Work out the finished part from the listing and answer in its coordinate system (mm). Face numbers are marked on the shaded views. A direction names the side the tool comes from. Coordinates: 2 decimals unless noted, no trailing zeros. Write each loop counter-clockwise with the first axis right and the second up, starting at its lowest first coordinate (ties: lowest second). Pieces come first, ordered by that corner, then holes. Notation, with made-up numbers: (22, 42.25) - (27, 42.25) arc R24 ccw to (27, 80.25) - close; hole circle Ø1 at (-8.5, -30.5). An arc over 180 degrees is marked (long way). One line per item, written item: value.
```python
from build123d import *

# Parameters (mm, degrees)
F1_DEPTH    = 8
F3_DEPTH    = 15
F4_T1_DEPTH = 8
F5_W        = 19.4
F5_H        = 25.4
F6_DEPTH    = 1.6
F7_W        = 17.4
F7_H        = 23.4
F8_DEPTH    = 25
F9_W        = 17.6963857411
F9_H        = 23.4
F10_DEPTH   = 5
F11_W       = 1
F11_H       = 16
F12_DEPTH   = 2


# Not quite as in the source:
# - a fillet or chamfer that OpenCascade refuses, or shapes differently, is made with other operations: its cross-section is extruded or revolved along the edge and cut away or added
# - a feature of the source that left no trace in its solid (it failed there, or was rolled back) is left out


with BuildPart() as f1:
    # F0 (on Front) → F1 (new body)
    with BuildSketch(Plane.XZ):
        with BuildLine():
            Line((5.123475383, -16.5), (14, -16.5))
            Line((14, -16.5), (14, 16.5))
            Line((14, 16.5), (5.123475383, 16.5))
            ThreePointArc((5.123475383, 16.5), (0, 14), (-5.123475383, 16.5))
            Line((-5.123475383, 16.5), (-14, 16.5))
            Line((-14, 16.5), (-14, -16.5))
            Line((-14, -16.5), (-5.123475383, -16.5))
            ThreePointArc((-5.123475383, -16.5), (0, -14), (5.123475383, -16.5))
        make_face()
    extrude(amount=F1_DEPTH)

    # F0 (on Front) → F3 (join)
    with BuildSketch(Plane.XZ):
        with BuildLine():
            ThreePointArc((6.5, -20.5), (6.1462423475, -18.3848865266), (5.123475383, -16.5))
            Line((5.123475383, -16.5), (1.4361406616, -16.5))
            ThreePointArc((1.4361406616, -16.5), (3.4760680238, -18.0547083826), (4.25, -20.5))
            ThreePointArc((4.25, -20.5), (-2.4452916174, -23.9760680238), (-1.4361406616, -16.5))
            Line((-1.4361406616, -16.5), (-5.123475383, -16.5))
            ThreePointArc((-5.123475383, -16.5), (-2.1151134734, -26.6462423475), (6.5, -20.5))
        make_face()
        with BuildLine():
            Line((1.4361406616, -16.5), (5.123475383, -16.5))
            ThreePointArc((5.123475383, -16.5), (0, -14), (-5.123475383, -16.5))
            Line((-5.123475383, -16.5), (-1.4361406616, -16.5))
            ThreePointArc((-1.4361406616, -16.5), (0, -16.25), (1.4361406616, -16.5))
        make_face()
        with BuildLine():
            ThreePointArc((-5.123475383, 16.5), (0, 14), (5.123475383, 16.5))
            Line((5.123475383, 16.5), (1.4361406616, 16.5))
            ThreePointArc((1.4361406616, 16.5), (0, 16.25), (-1.4361406616, 16.5))
            Line((-1.4361406616, 16.5), (-5.123475383, 16.5))
        make_face()
        with BuildLine():
            Line((1.4361406616, 16.5), (5.123475383, 16.5))
            ThreePointArc((5.123475383, 16.5), (6.1462423475, 18.3848865266), (6.5, 20.5))
            ThreePointArc((6.5, 20.5), (-2.1151134734, 26.6462423475), (-5.123475383, 16.5))
            Line((-5.123475383, 16.5), (-1.4361406616, 16.5))
            ThreePointArc((-1.4361406616, 16.5), (-2.4452916174, 23.9760680238), (4.25, 20.5))
            ThreePointArc((4.25, 20.5), (3.4760680238, 18.0547083826), (1.4361406616, 16.5))
        make_face()
    extrude(amount=F3_DEPTH)

    # F4: chamfer of 1.9 on 4 edges, made by hand

    # F4_s2 → F4_t1 (join)
    with BuildSketch(Plane.XZ):
        with BuildLine():
            Line((-6.8027454264, 16.4361025598), (-5.876418772, 17.87458352))
            Line((-5.876418772, 17.87458352), (-5.8418237692, 17.8903056629))
            ThreePointArc((-5.8418237692, 17.8903056629), (-5.5354543935, 17.1659051218), (-5.0935227577, 16.5233846154))
            Line((-5.0935227577, 16.5233846154), (-5.123475383, 16.462))
            ThreePointArc((-5.123475383, 16.462), (-5.9631104047, 16.462), (-6.8027454264, 16.3981025598))
            Line((-6.8027454264, 16.3981025598), (-6.8027454264, 16.4361025598))
        make_face()
        with BuildLine():
            Line((5.876418772, 17.87458352), (6.8027454264, 16.4361025598))
            Line((6.8027454264, 16.4361025598), (6.8027454264, 16.3981025598))
            ThreePointArc((6.8027454264, 16.3981025598), (5.9631104047, 16.462), (5.123475383, 16.462))
            Line((5.123475383, 16.462), (5.0935227577, 16.5233846154))
            ThreePointArc((5.0935227577, 16.5233846154), (5.5354543935, 17.1659051218), (5.8418237692, 17.8903056629))
            Line((5.8418237692, 17.8903056629), (5.876418772, 17.87458352))
        make_face()
        with BuildLine():
            Line((6.8027454264, -16.4361025598), (5.876418772, -17.87458352))
            Line((5.876418772, -17.87458352), (5.8418237692, -17.8903056629))
            ThreePointArc((5.8418237692, -17.8903056629), (5.5354543935, -17.1659051218), (5.0935227577, -16.5233846154))
            Line((5.0935227577, -16.5233846154), (5.123475383, -16.462))
            ThreePointArc((5.123475383, -16.462), (5.9631104047, -16.462), (6.8027454264, -16.3981025598))
            Line((6.8027454264, -16.3981025598), (6.8027454264, -16.4361025598))
        make_face()
        with BuildLine():
            Line((-6.8027454264, -16.4361025598), (-5.876418772, -17.87458352))
            Line((-5.876418772, -17.87458352), (-5.8418237692, -17.8903056629))
            ThreePointArc((-5.8418237692, -17.8903056629), (-5.5354543935, -17.1659051218), (-5.0935227577, -16.5233846154))
            Line((-5.0935227577, -16.5233846154), (-5.123475383, -16.462))
            ThreePointArc((-5.123475383, -16.462), (-5.9631104047, -16.462), (-6.8027454264, -16.3981025598))
            Line((-6.8027454264, -16.3981025598), (-6.8027454264, -16.4361025598))
        make_face()
    extrude(amount=F4_T1_DEPTH)

    # F5 (on face) → F6 (cut)
    with BuildSketch(Plane.XZ.offset(8)):
        with Locations((2.3, 0)):
            Rectangle(F5_W, F5_H)
    extrude(amount=-F6_DEPTH, mode=Mode.SUBTRACT)

    # F7 (on face) → F8 (cut)
    with BuildSketch(Plane.XZ.offset(6.4)):
        with Locations((2.3, 0)):
            Rectangle(F7_W, F7_H)
    extrude(amount=-F8_DEPTH, mode=Mode.SUBTRACT)

    # F9 (on face) → F10 (cut)
    with BuildSketch(Plane.XZ):
        with Locations((-5.1518071295, 0)):
            Rectangle(F9_W, F9_H)
    extrude(amount=F10_DEPTH, mode=Mode.SUBTRACT)

    # F11 (on face) → F12 (cut)
    with BuildSketch(Plane.XZ.offset(6.4)):
        with Locations((11.5, 0.4684822634)):
            Rectangle(F11_W, F11_H)
    extrude(amount=-F12_DEPTH, mode=Mode.SUBTRACT)


solid = f1.part
```
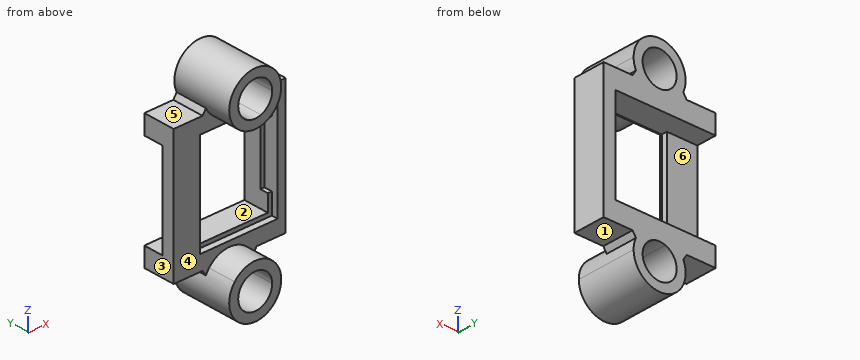
Item 1: Section B-B, the plane y = -12.5 is taken. Determine the outline of the cut face in (x, z).
Evaluation:
outline: circle Ø13 at (0, -20.5); circle Ø13 at (0, 20.5); hole circle Ø8.5 at (0, -20.5); hole circle Ø8.5 at (0, 20.5)
Item 2: Determine the mould class of the marked faces 1, 2 and 3 for opening direction X: +X half, -X half, draft (parallel to the pull), parting line (faces both ways), or undercut.
Evaluation:
face 1: draft
face 2: undercut
face 3: -X half
Item 3: Which of the six approach directions +Z, -Z, +X, -X, +Y, -Y give full straight-line access (tool end or side, diameter ignored) to the marked faces 4, 5 and 6?
Evaluation:
face 4: -Y
face 5: +Z, -X, +Y, -Y
face 6: -X, +Y
Item 4: Consider probe 1 along Z at (x, y) = (0, -6.5); probe 2 along X at (y, z) = (-8.5, -20.5); probe 3 along Z at (x, y) = (-3, -1). Determine where each line is inside the solid, lowest interval first.
Evaluation:
probe 1: z = -27 to -24.75, -16.25 to -12.7, 12.7 to 16.25, 24.75 to 27
probe 2: x = -6.5 to -4.25, 4.25 to 6.5
probe 3: z = -26.27 to -23.51, -17.49 to -11.7, 11.7 to 17.49, 23.51 to 26.27
Item 5: Section C-C, the plane x = 0 is taken. Determine the outline of the cut face in (y, z), then the cut area to 3 significant figures.
Evaluation:
outline: (-15, -27) - (0, -27) - (0, -24.75) - (-15, -24.75) - close; (-15, -16.25) - (0, -16.25) - (0, -11.7) - (-6.4, -11.7) - (-6.4, -12.7) - (-8, -12.7) - (-8, -14) - (-15, -14) - close; (-15, 14) - (-8, 14) - (-8, 12.7) - (-6.4, 12.7) - (-6.4, 11.7) - (0, 11.7) - (0, 16.25) - (-15, 16.25) - close; (-15, 24.75) - (0, 24.75) - (0, 27) - (-15, 27) - close
area: 169 mm2
Item 6: Given pin 1 (2 mm diameter, centred on x = -10.5, y = -5, fed in from +Z); pin 2 (2 mm diameter, centred on y = -6, z = 21.5, fed in from -X); pin 3 (1 mm diameter, centred on y = -9.5, z = 17, fed in from +X); pin 4 (3 mm diameter, centred on y = -11, z = 1, fed in from -X), each flat-ended and moving along its own axis, determine where each tip first touches the part or whether it passes through.
Evaluation:
pin 1: stops at z = 16.5
pin 2: stops at x = -6.5
pin 3: stops at x = 5.77
pin 4: passes through
Item 7: Section A-A, the plane z = 3 is taken. Determine the outline of the cut face in (x, y), then the cut area to 3 significant figures.
Evaluation:
outline: (-14, -8) - (-7.4, -8) - (-7.4, -6.4) - (-6.4, -6.4) - (-6.4, -5) - (-14, -5) - close; (11, -4.4) - (12, -4.4) - (12, -8) - (14, -8) - (14, 0) - (11, 0) - close
area: 41.6 mm2
Item 8: Section D-D, the plane y = -3.25 is taken. Determine the outline of the cut face in (x, z).
Evaluation:
outline: (-14, -16.5) - (-6.76, -16.5) - (-5.92, -17.81) arc R6.5 ccw (long way) to (5.92, -17.81) - (6.76, -16.5) - (14, -16.5) - (14, 16.5) - (6.76, 16.5) - (5.92, 17.81) arc R6.5 ccw (long way) to (-5.92, 17.81) - (-6.76, 16.5) - (-14, 16.5) - (-14, 11.7) - (11, 11.7) - (11, -11.7) - (-14, -11.7) - close; hole circle Ø8.5 at (0, -20.5); hole circle Ø8.5 at (0, 20.5)
